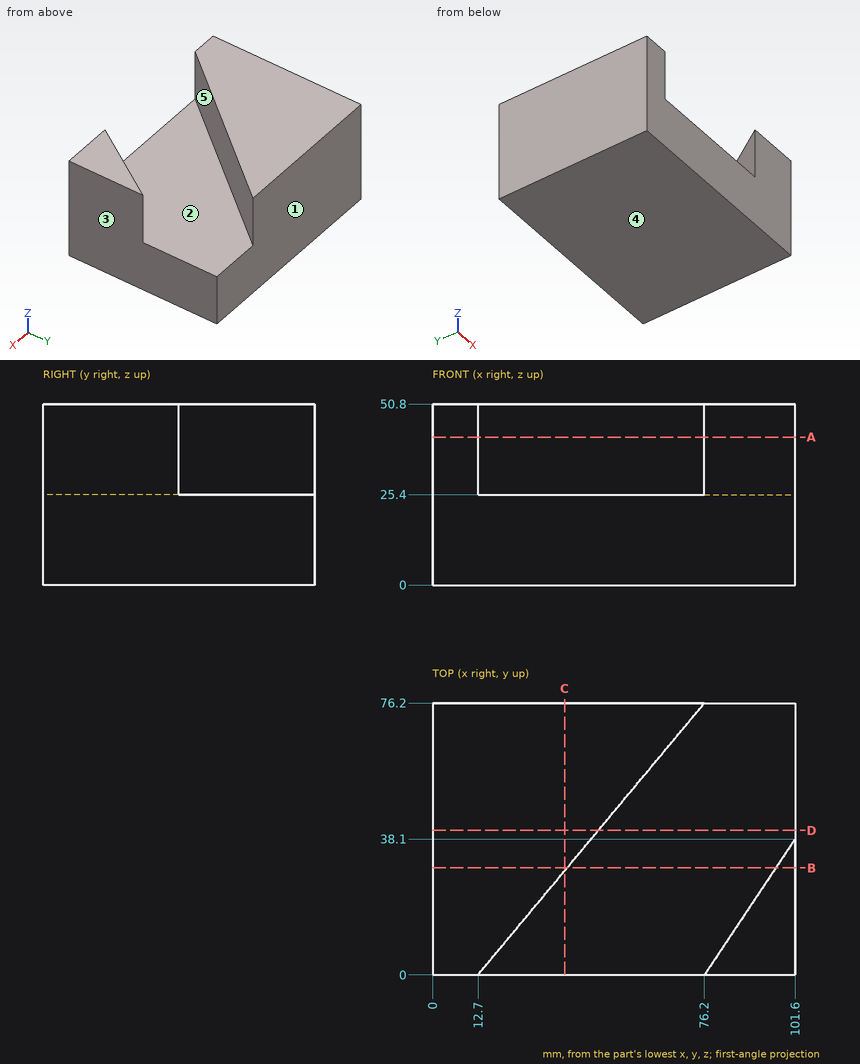
Design review of the part shown in the three views and the two pictorial views. Dimensions are in mm from the part's minimum x, y and z. A direction names the side the tool comes from. Round coordinates to 2 decimals unless told otherwise and drop trailing zeros. Loops run counter-clockwise (first coordinate to the right, second up) from the corner with the lowest first, then second, coordinate; pieces in that order, holes last. Notation, with made-up numbers: (10.25, 1) - (23.25, 1) arc R34 ccw to (23.25, 38) - close; hole circle Ø10 at (66, 89). An arc over 180 degrees is marked (long way). Use one line per item in the form item = value.
1) Mouldability with a two-part tool opening along X and no side actions: class the marked faces 1, 2 and 3 as pulls with the +X half, pulls with the -X half, needs draft (parallel to the pull), parting line crosses it, or undercut.
Solutions:
face_1 = needs draft
face_2 = undercut
face_3 = pulls with the +X half
2) Wall thickness on probe 1 along Z at (x, y) = (81.5, 13.5); probe 2 along X at (y, z) = (14, 46); probe 3 along X at (y, z) = (31, 38.5): over which ranges is each line inside the solid? List them lowest first.
Solutions:
probe_1 = 0 to 25.4
probe_2 = 0 to 24.37, 85.53 to 101.6
probe_3 = 0 to 38.53, 96.87 to 101.6
3) We need section D-D on y = 40.5. Write out the cut boundary in (x, z), then the cut area to 3 significant figures.
Solutions:
outline = (0, 0) - (101.6, 0) - (101.6, 25.4) - (46.45, 25.4) - (46.45, 50.8) - (0, 50.8) - close
area = 3,760 mm2
4) We need section B-B on y = 30. Write out the cut boundary in (x, z).
Solutions:
outline = (0, 0) - (101.6, 0) - (101.6, 50.8) - (96.2, 50.8) - (96.2, 25.4) - (37.7, 25.4) - (37.7, 50.8) - (0, 50.8) - close
5) Clearance check with a flat-ended pin moving along its axis: P1, Ø6, axis at x = 49.5, y = 34.5, coming from the +Z side. State where the tip first meets the part, or that it passes through.
Solutions:
P1 = 25.4
6) We need section C-C on x = 37. Write out the cut boundary in (y, z), then the cut area to 3 significant figures.
Solutions:
outline = (0, 0) - (76.2, 0) - (76.2, 50.8) - (29.16, 50.8) - (29.16, 25.4) - (0, 25.4) - close
area = 3,130 mm2
7) Tool access review of the marked faces 4 and 5: name each direction out of +Z, -Z, +X, -X, +Y, -Y from which nothing blocks a thin tool from reaching the whole face with its end or side.
Solutions:
face_4 = -Z, +X, -X, +Y, -Y
face_5 = +Z, -Y
8) We need section A-A on z = 41.5. Write out the cut boundary in (x, y), then the cut area to 3 significant figures.
Solutions:
outline = (0, 0) - (12.7, 0) - (76.2, 76.2) - (0, 76.2) - close; (76.2, 0) - (101.6, 0) - (101.6, 38.1) - close
area = 3,870 mm2
